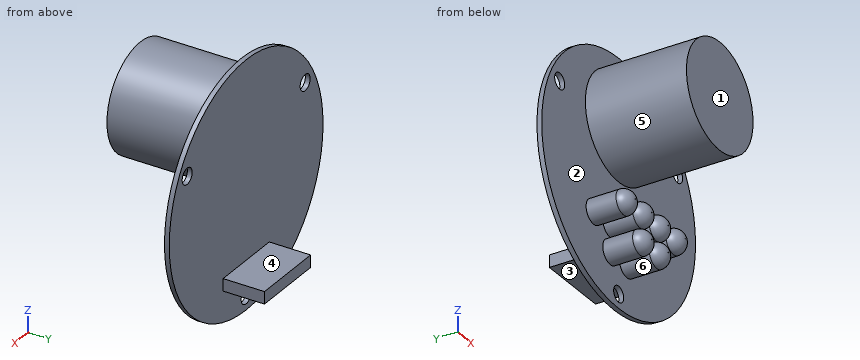
```python
from build123d import *

# Parameters (mm, degrees)
F0_R      = 25.4
F1_DEPTH  = 1
F2_R      = 1.65
F3_DEPTH  = 1.001
F4_R      = 11
F5_DEPTH  = 21
F6_R      = 2.5
F7_DEPTH  = 8.6
F8_R      = 2.4
F9_W      = 15.24
F9_H      = 2.54
F10_DEPTH = 8.6


with BuildPart() as f1:
    # F0 (on Front) → F1 (new body)
    with BuildSketch(Plane.XZ):
        Circle(F0_R)
    extrude(amount=F1_DEPTH)

    # F2 (on face) → F3 (cut, through all)
    with BuildSketch(Plane.XZ.offset(1)):
        with Locations((-19.485572, 11.25)):
            Circle(F2_R)
        with Locations((0, -22.5)):
            Circle(F2_R)
        with Locations((19.485572, 11.25)):
            Circle(F2_R)
    extrude(amount=-F3_DEPTH, mode=Mode.SUBTRACT)

    # F4 (on face) → F5 (join)
    with BuildSketch(Plane.XZ.offset(1)):
        with Locations((0, 11.25)):
            Circle(F4_R)
    extrude(amount=F5_DEPTH)

    # F6 (on face) → F7 (join)
    with BuildSketch(Plane.XZ.offset(1)):
        with Locations((-8.25, -9.85)):
            Circle(F6_R)
        with Locations((-2.75, -15.35)):
            Circle(F6_R)
        with Locations((-2.75, -9.85)):
            Circle(F6_R)
        with Locations((2.75, -15.35)):
            Circle(F6_R)
        with Locations((8.25, -9.85)):
            Circle(F6_R)
        with Locations((2.75, -9.85)):
            Circle(F6_R)
    extrude(amount=F7_DEPTH)

    # F8
    f8_edges = [f1.edges().sort_by_distance(p)[0] for p in [
        (-10.75, -9.6, -9.85),
        (-5.25, -9.6, -9.85),
        (0.25, -9.6, -9.85),
        (5.75, -9.6, -9.85),
        (0.25, -9.6, -15.35),
        (-5.25, -9.6, -15.35),
    ]]
    fillet(f8_edges, radius=F8_R)

    # F9 (on face) → F10 (join)
    with BuildSketch(Plane(origin=(0, 0, 0), x_dir=(-1, 0, 0), z_dir=(0, 1, 0))):
        with Locations((0, -16.58)):
            Rectangle(F9_W, F9_H)
    extrude(amount=F10_DEPTH)


solid = f1.part
```
Model file for the job. Use its own axes, mm. Face numbers are marked on the shaded views. A direction names the side the tool comes from. Round coordinates to 2 decimals unless told otherwise and drop trailing zeros. Loops run counter-clockwise (first coordinate to the right, second up) from the corner with the lowest first, then second, coordinate; pieces in that order, holes last. Notation, with made-up numbers: M 39.25,60 L 52.25,60 A30 ccw 52.25,98 Z; hole C 68,75.25 d9. An arc over 180 degrees is marked long. Put each result on its own line as item: value. Start each with the question number.
Item 1: Cut at C-C (y = -19). List the corners of the cut face in (x, z).
Item 2: 3-axis set-ups, long thin cutter, end or side, ignore diameter. For the marked faces 1, 2 and 3: which of +Z, -Z, +X, -X, +Y, -Y reach the whole face in a straight line?
Item 3: Cut at D-D (x = -16.5). List the corners of the cut face in (y, z).
Item 4: Mould opens along X. For the marked faces 4, 5 and 6 say: released by +X, released by -X, zero draft, split by the parting line, or undercut.
Item 5: Cut at B-B (z = 21). List the corners of the cut face in (x, y).
Item 6: Cut at A-A (z = -22.5). List the corners of the cut face in (x, y), then the cut area to 3 significant figures.
Item 7: Drop flat-ended pins along their axis: P1, Ø1.5, axis at y = -14, z = 8.5, coming from the +X side; P2, Ø10, axis at x = 7, y = -6.5, coming from the +Z side; P3, Ø6, axis at x = -16.5, z = 9, coming from the +Y side. Give the stop position or say it passes through.
Item 8: Drill centre lines: line 1 along Z through (x, y) = (0, -0.6); line 2 along Z through (x, y) = (3, -9); line 3 along Y through (x, z) = (11.5, -3). Where is each one in solid material? Low to high.
Answer block:
1. outline: C 0,11.25 d22
2. face 1: +Z, -Z, +X, -X, -Y
2. face 2: -Y
2. face 3: -Z, +X, -X, +Y
3. outline: M -1,-19.31 L 0,-19.31 L 0,19.31 L -1,19.31 Z
4. face 4: zero draft
4. face 5: split by the parting line
4. face 6: undercut
5. outline: M -14.29,-1 L -5.09,-1 L -5.09,-22 L 5.09,-22 L 5.09,-1 L 14.29,-1 L 14.29,0 L -14.29,0 Z
6. outline: M -11.79,-1 L -1.65,-1 L -1.65,0 L -11.79,0 Z; M 1.65,-1 L 11.79,-1 L 11.79,0 L 1.65,0 Z
6. area: 20.3 mm2
7. P1: x = 10.82
7. P2: z = 22.07
7. P3: y = 0
8. line 1: -25.4 to -24.15, -20.85 to 25.4
8. line 2: -17.02 to -13.68, -11.52 to -8.18, 0.67 to 21.83
8. line 3: -1 to 0
